Source: CAD feature listing. Evaluate the final solid. Frame: model axes, mm. A direction names the side the tool comes from. Give positions to 0.01 mm unless a question says otherwise; leave off trailing zeros. Order: outer loops, then holes, each group sorted by start corner. A loop starts at its lowest first (then second) coordinate and runs counter-clockwise, first axis right, second up.
Autodesk Inventor part; units mm, degrees
ref_plane "YZ Plane" through (0, 0, 0) normal (1, 0, 0) x (0, 1, 0)
ref_plane "XZ Plane" through (0, 0, 0) normal (0, 1, 0) x (-1, 0, 0)
ref_plane "XY Plane" through (0, 0, 0) normal (0, 0, 1) x (1, 0, 0)
sketch "Skizze1" plane through (0, 0, 0) normal (0, 0, 1) x (1, 0, 0)
  line L0 (0, 16.1) -> (0, -16.1)
  line L1 (-8.4, 0) -> (8.4, 0)
  line L2 (-6, -11.5) -> (6, -11.5)
  line L3 (6, -11.5) -> (6, 11.5)
  line L4 (6, 11.5) -> (-6, 11.5)
  line L5 (-6, 11.5) -> (-6, -11.5)
  line L6 (-6, -11.5) -> (6, 11.5) construction
  line L7 (6, -11.5) -> (-6, 11.5) construction
  point P0 (0, 0)
  dimension "d0" = 12
  dimension "d1" = 23
extrude "Extrusion1" add sketch "Skizze1" along normal blind 16.2
sketch "Skizze2" plane through (0, 0, 16.2) normal (0, 0, 1) x (1, 0, 0)
  line L0 (-6, -11.5) -> (-6, 11.5)
  line L1 (-6, 11.5) -> (6, 11.5)
  line L2 (6, 11.5) -> (6, -11.5)
  line L3 (6, -11.5) -> (-6, -11.5)
  line L4 (6, 11.5) -> (-6, 11.5)
  line L5 (-6, 11.5) -> (-6, 16.5)
  line L6 (-6, 16.5) -> (6, 16.5)
  line L7 (6, 16.5) -> (6, 11.5)
  line L8 (-6, -11.5) -> (6, -11.5)
  line L9 (6, -11.5) -> (6, -16.5)
  line L10 (6, -16.5) -> (-6, -16.5)
  line L11 (-6, -16.5) -> (-6, -11.5)
  line L12 (-6, 11.5) -> (-6, -11.5)
  point P0 (0, 0)
  dimension "d4" = 5
  dimension "d5" = 5
extrude "Extrusion2" add sketch "Skizze2" along normal blind 2.3
sketch "Skizze3" plane through (0, 0, 18.5) normal (0, 0, 1) x (1, 0, 0)
  line L0 (6, -16.5) -> (-6, -16.5)
  line L1 (-6, -16.5) -> (-6, 16.5)
  line L2 (-6, 16.5) -> (6, 16.5)
  line L3 (6, 16.5) -> (6, -16.5)
  line L4 (-6, -11.5) -> (6, -11.5)
  line L5 (6, -11.5) -> (6, 11.5)
  line L6 (6, 11.5) -> (-6, 11.5)
  line L7 (-6, 11.5) -> (-6, -11.5)
  line L8 (-6, -11.5) -> (6, 11.5) construction
  line L9 (6, -11.5) -> (-6, 11.5) construction
  point P0 (0, 0)
  dimension "d8" = 11.5
extrude "Extrusion3" add sketch "Skizze3" along normal blind 4.5 contours L4 L1 L6 L3
sketch "Skizze4" plane through (0, 0, 23) normal (0, 0, 1) x (1, 0, 0)
  line L0 (-6, 11.5) -> (6, 11.5)
  line L1 (6, 11.5) -> (6, -11.5)
  line L2 (6, -11.5) -> (-6, -11.5)
  line L3 (-6, -11.5) -> (-6, 11.5)
  line L4 (6, 16.5) -> (-6, 16.5)
  line L5 (-6, 16.5) -> (-6, 11.5)
  line L6 (6, 11.5) -> (6, 16.5)
  line L7 (6, -16.5) -> (6, -11.5)
  line L8 (-6, -16.5) -> (6, -16.5)
  line L9 (-6, -11.5) -> (-6, -16.5)
  line L10 (-8.4, 0) -> (8.4, 0)
  line L11 (0, 23.1) -> (0, -23.1)
  circle A0 centre (0, 5.5) radius 6
  circle A1 centre (0, -0.5) radius 3
  point P0 (0, 0)
  dimension "d11" = 11
  dimension "d12" = 12
  dimension "d13" = 17
  dimension "d14" = 6
extrude "Extrusion4" add sketch "Skizze4" along normal blind 4.1 contours A0 A1 L11 | L11 A1 A0 | A1 A0 L10 L11 | L11 L10 A0 A1 | A0 L10 A1 | L11 A0 L10 | L10 A0 L11 | A1 L10 A0 | L10 A0 L11 A1 | L10 A1 L11 A0
sketch "Skizze5" plane through (0, 0, 27.1) normal (0, 0, 1) x (1, 0, 0)
  arc A0 (2.9047, 0.25) -> (-2.9047, 0.25) centre (0, 5.5) ccw
  arc A1 (-2.9047, 0.25) -> (2.9047, 0.25) centre (0, -0.5) ccw
  circle A2 centre (0, 5.5) radius 2.4
  point P0 (0, 0)
  dimension "d17" = 4.8
extrude "Extrusion5" add sketch "Skizze5" along normal blind 2.8 contours A2
sketch "Skizze6" plane through (0, 0, 18.5) normal (0, 0, 1) x (1, 0, 0)
  line L0 (6, -16.5) -> (-6, -16.5)
  line L1 (-6, -16.5) -> (-6, -11.5)
  line L2 (6, -11.5) -> (-6, -11.5)
  line L3 (6, 11.5) -> (6, -11.5)
  line L4 (-6, 11.5) -> (6, 11.5)
  line L5 (-6, 11.5) -> (-6, 16.5)
  line L6 (-6, 16.5) -> (6, 16.5)
  line L7 (6, 16.5) -> (6, 11.5)
  line L8 (6, -11.5) -> (6, -16.5)
  line L9 (-6, -11.5) -> (-6, 11.5)
  line L10 (0, 23.1) -> (0, -23.1)
  circle A0 centre (0, 14.2) radius 1.1
  line L11 (6, 16.5) -> (-6, 16.5)
  line L12 (0.6, 14.1) -> (-0.6, 14.1)
  line L13 (-0.6, 14.1) -> (-0.6, 16.5)
  line L14 (-0.6, 16.5) -> (0.6, 16.5)
  line L15 (0.6, 16.5) -> (0.6, 14.1)
  line L16 (0.6, 14.1) -> (-0.6, 16.5) construction
  line L17 (-0.6, 14.1) -> (0.6, 16.5) construction
  point P0 (0, 0)
  point P1 (0, 15.3)
  dimension "d21" = 2.2
  dimension "d20" = 2.3
  dimension "d22" = 1.2
extrude "Extrusion6" cut sketch "Skizze6" against normal blind 2.8 contours A0 L13 L12 L10 | L10 L12 L15 A0 | L15 A0 L10 L6 | L12 L13 A0 L10 | L10 A0 L15 L12 | L13 L6 L10 A0
mirror "Spiegeln1" about plane through (0, 0, 0) normal (0, 1, 0) of "Extrusion6"
properties part number "Mikroservo" material "ABS-Kunststoff"
1) Section query B-B, the plane y = -0.5. Return the cut outline in (x, z), and give its area (3 significant figures).
Report:
outline: (-6, 0) - (6, 0) - (6, 23) - (3, 23) - (3, 27.1) - (-3, 27.1) - (-3, 23) - (-6, 23) - close
area: 301 mm2
2) Material intervals for L1, parallel to X at y = -14.2, z = 17.7; L2, parallel to Y at x = 0, z = 16.8; L3, parallel to Y at x = -3, z = 1.75, sorted ascending.
Report:
L1: x = -6 to -1.1, 1.1 to 6
L2: y = -13.1 to 13.1
L3: y = -11.5 to 11.5
3) Section query D-D, the plane z = 5.5. Return the cut outline in (x, y).
Report:
outline: (-6, -11.5) - (6, -11.5) - (6, 11.5) - (-6, 11.5) - close
4) Section query A-A, the plane y = -14.2. Return the cut outline in (x, z).
Report:
outline: (-6, 16.2) - (-1.1, 16.2) - (-1.1, 18.5) - (-6, 18.5) - close; (1.1, 16.2) - (6, 16.2) - (6, 18.5) - (1.1, 18.5) - close
5) Reachability of faces 4 (the cylindrical face through (0.1, -3.5, 25)), 5 (the flat face through (-0.6, -16, 17)), 6 (the flat face through (0, 11.5, 21)), 7 (the flat face through (0, 11.5, 8)) from +Z, -Z, +X, -X, +Y, -Y: full face, straight path, thin tool, end or side. Return the list, or none.
Report:
face 4: +Z
face 5: +Z, -Z, -Y
face 6: +Z, +X, -X, +Y
face 7: -Z, +X, -X, +Y
6) Section query C-C, the plane x = -3.5. Return the cut outline in (y, z).
Report:
outline: (-16.5, 16.2) - (-11.5, 16.2) - (-11.5, 0) - (11.5, 0) - (11.5, 16.2) - (16.5, 16.2) - (16.5, 18.5) - (11.5, 18.5) - (11.5, 23) - (10.37, 23) - (10.37, 27.1) - (0.63, 27.1) - (0.63, 23) - (-11.5, 23) - (-11.5, 18.5) - (-16.5, 18.5) - close
7) Pin query (flat end, axial travel): pin 1 (1.5 mm diameter, centred on x = 2, z = 24, fed in from +Y); pin 2 (2.5 mm diameter, centred on x = -2, y = 14.5, fed in from +Z); pin 3 (5 mm diameter, centred on x = -2, z = 21.5, fed in from +Y); pin 4 (1.8 mm diameter, centred on x = 0, y = 14.2, fed in from -Z). Return the tip coordinate at first contact, or that it passes through.
Report:
pin 1: stops at y = 11.37
pin 2: stops at z = 18.5
pin 3: stops at y = 11.5
pin 4: passes through
8) Draft query along Y for faces 1 (the flat face through (-0.1, 12.9, 18.5)), 2 (the cylindrical face through (1.29, 3.476, 28.48)), 3 (the cylindrical face through (0, 13.1, 17.4)). Return one class per face: +Y half, -Y half, draft (parallel to the pull), parting line (faces both ways), or undercut.
Report:
face 1: draft
face 2: parting line
face 3: undercut
